Design review of the part built by this model. Coordinates are the model's own, in mm. Coordinates: 2 decimals unless noted, no trailing zeros. Write each loop counter-clockwise with the first axis right and the second up, starting at its lowest first coordinate (ties: lowest second). Pieces come first, ordered by that corner, then holes. Notation, with made-up numbers: (65, 23.25) - (79, 23.25) arc R16 ccw to (79, 40.25) - close; hole circle Ø7 at (33.5, 69). An arc over 180 degrees is marked (long way). Use a Markdown table: item, result.
Autodesk Inventor part; units mm, degrees
ref_plane "tuer_XY" through (241.2, -320.6, -8.2) normal (0, 1, 0) x (1, 0, 0)
ref_plane "tuer_YZ" through (241.2, -320.6, -8.2) normal (1, 0, 0) x (0, 0, -1)
ref_plane "tuer_ZX" through (241.2, -320.6, -8.2) normal (0, 0, -1) x (0, 1, 0)
sketch "Skizze_1" plane through (0, 0, 0) normal (0, 0, 1) x (1, 0, 0)
  line L0 (-247.5, 377.5) -> (-247.5, -377.5)
  line L1 (-247.5, -377.5) -> (247.5, -377.5)
  line L2 (247.5, -377.5) -> (247.5, 377.5)
  line L3 (247.5, 377.5) -> (-247.5, 377.5)
extrude "Extrusion1" add sketch "Skizze_1" against normal blind 15
sketch "Skizze_2" plane through (0, 0, 0) normal (1, 0, 0) x (0, 0, -1)
  line L0 (2, 375.5) -> (2, -375.5)
  line L1 (2, -375.5) -> (17, -375.5)
  line L2 (17, -375.5) -> (17, 375.5)
  line L3 (17, 375.5) -> (2, 375.5)
extrude "Extrusion2" cut sketch "Skizze_2" along normal mid plane 491
sketch "Skizze_3" plane through (0, 0, -2) normal (0, 0, 1) x (1, 0, 0)
  line L0 (-245.5, 361.5) -> (231.5, 361.5)
  line L1 (231.5, 361.5) -> (231.5, -361.5)
  line L2 (231.5, -361.5) -> (-245.5, -361.5)
  line L3 (-245.5, -361.5) -> (-245.5, -373.5)
  line L4 (-245.5, -373.5) -> (243.5, -373.5)
  line L5 (243.5, -373.5) -> (243.5, 373.5)
  line L6 (243.5, 373.5) -> (-245.5, 373.5)
  line L7 (-245.5, 373.5) -> (-245.5, 361.5)
sketch "Skizze_21" plane through (0, -320.6, 0) normal (0, 1, 0) x (1, 0, 0)
  arc A0 (241.2, 12.35) -> (241.2, 4.05) centre (241.2, 8.2) ccw
  line L0 (241.2, 4.05) -> (245.5, 4.05)
  line L1 (245.5, 4.05) -> (245.5, 5.5)
  line L2 (245.5, 5.5) -> (241.2, 5.5)
  arc A1 (241.2, 10.9) -> (241.2, 5.5) centre (241.2, 8.2) ccw
  line L3 (241.2, 10.9) -> (245.5, 10.9)
  line L4 (245.5, 10.9) -> (245.5, 12.35)
  line L5 (245.5, 12.35) -> (241.2, 12.35)
extrude "Extrusion3" add sketch "Skizze_21" along normal mid plane 26
sketch "Skizze_22" plane through (0, 320.6, 0) normal (0, 1, 0) x (1, 0, 0)
  arc A0 (241.2, 12.35) -> (241.2, 4.05) centre (241.2, 8.2) ccw
  line L0 (241.2, 4.05) -> (245.5, 4.05)
  line L1 (245.5, 4.05) -> (245.5, 5.5)
  line L2 (245.5, 5.5) -> (241.2, 5.5)
  arc A1 (241.2, 10.9) -> (241.2, 5.5) centre (241.2, 8.2) ccw
  line L3 (241.2, 10.9) -> (245.5, 10.9)
  line L4 (245.5, 10.9) -> (245.5, 12.35)
  line L5 (245.5, 12.35) -> (241.2, 12.35)
extrude "Extrusion4" add sketch "Skizze_22" along normal mid plane 26
sketch "Skizze_24" plane through (0, 0, 0) normal (0, 0, 1) x (1, 0, 0)
  line L0 (-221.05, -318.95) -> (-221.05, -341.05)
  line L1 (-221.05, -341.05) -> (-198.95, -341.05)
  line L2 (-198.95, -341.05) -> (-198.95, -318.95)
  line L3 (-198.95, -318.95) -> (-221.05, -318.95)
extrude "Extrusion5" cut sketch "Skizze_24" against normal blind 2
sketch "Skizze_41" plane through (0, 0, 0) normal (0, 0, 1) x (1, 0, 0)
  line L0 (-221.05, 341.05) -> (-221.05, 318.95)
  line L1 (-221.05, 318.95) -> (-198.95, 318.95)
  line L2 (-198.95, 318.95) -> (-198.95, 341.05)
  line L3 (-198.95, 341.05) -> (-221.05, 341.05)
extrude "Extrusion6" cut sketch "Skizze_41" against normal blind 2
sketch "Skizze_23" plane through (-247.5, 0, 0) normal (1, 0, 0) x (0, 0, -1)
  arc A0 (13.25, 372.2142) -> (13.25, 354.7858) centre (15.5, 363.5) ccw
  arc A1 (15.5, 351.881) -> (13.25, 354.7858) centre (12.5, 351.881) ccw
  line L0 (15.5, 351.881) -> (15.5, 375.119)
  arc A2 (13.25, 372.2142) -> (15.5, 375.119) centre (12.5, 375.119) ccw
extrude "Extrusion7" cut sketch "Skizze_23" along normal blind 3
sketch "Skizze_26" plane through (-247.5, 0, 0) normal (1, 0, 0) x (0, 0, -1)
  arc A0 (13.25, -354.7858) -> (13.25, -372.2142) centre (15.5, -363.5) ccw
  arc A1 (15.5, -375.119) -> (13.25, -372.2142) centre (12.5, -375.119) ccw
  line L0 (15.5, -375.119) -> (15.5, -351.881)
  arc A2 (13.25, -354.7858) -> (15.5, -351.881) centre (12.5, -351.881) ccw
extrude "Extrusion8" cut sketch "Skizze_26" along normal blind 3
extrude "Extrusion9" add sketch "Skizze_3" against normal blind 6.5
ref_plane "tuer_XY" through (241.2, -320.6, -8.2) normal (0, 1, 0) x (1, 0, 0)
ref_plane "tuer_YZ" through (241.2, -320.6, -8.2) normal (1, 0, 0) x (0, 0, -1)
ref_plane "tuer_ZX" through (241.2, -320.6, -8.2) normal (0, 0, -1) x (0, 1, 0)
ref_plane "verschluss_XY" through (-210, -330, 0) normal (0, 0, 1) x (1, 0, 0)
ref_plane "verschluss_YZ" through (-210, -330, 0) normal (1, 0, 0) x (0, 1, 0)
ref_plane "verschluss_ZX" through (-210, -330, 0) normal (0, 1, 0) x (0, 0, 1)
ref_plane "verschluss2_XY" through (-210, 330, 0) normal (0, 0, 1) x (1, 0, 0)
ref_plane "verschluss2_YZ" through (-210, 330, 0) normal (1, 0, 0) x (0, 1, 0)
ref_plane "verschluss2_ZX" through (-210, 330, 0) normal (0, 1, 0) x (0, 0, 1)
sketch "Эскиз10" plane through (0, 0, 0) normal (0, 0, 1) x (1, 0, 0)
  line L0 (-39.5, 292.5) -> (52.5, 292.5)
  line L1 (52.5, 292.5) -> (52.5, 200.5)
  line L2 (52.5, 200.5) -> (-39.5, 200.5)
  line L3 (-39.5, 200.5) -> (-39.5, 292.5)
  line L4 (247.5, -377.5) -> (247.5, 377.5)
  line L5 (247.5, 377.5) -> (-247.5, 377.5)
  point P0 (0, 0)
  dimension "d20" = 92
  dimension "d21" = 92
  dimension "d22" = 195
  dimension "d23" = 85
extrude "Выдавливание10" cut sketch "Эскиз10" against normal blind 10
properties part number "1130_01_03 (2)"
(1) For pin 1 (4 mm diameter, centred on x = 147, y = 268.5, fed in from -Z), flat-tipped, find the tip position at first contact; note if it passes through.
Determined:
| item | result |
|---|---|
| pin 1 | z = -2 |
(2) Take a section at B-B on y = -123.5. Write out the cut boundary in (x, z).
Determined:
| item | result |
|---|---|
| outline | (-247.5, -15) - (-245.5, -15) - (-245.5, -2) - (231.5, -2) - (231.5, -8.5) - (243.5, -8.5) - (243.5, -2) - (245.5, -2) - (245.5, -15) - (247.5, -15) - (247.5, 0) - (-247.5, 0) - close |
(3) Draft analysis for pull direction Y (two halves, no side actions). For faces 1 (the flat face through (3, 377.5, -7)), 2 (the flat face through (-10, 5, -2)), 3 (the flat face through (-3, -377.5, -7)), 4 (the flat face through (-3, 5, 0)), state which applies: +Y half, -Y half, draft (parallel to the pull), parting line (faces both ways), or undercut.
Determined:
| item | result |
|---|---|
| face 1 | +Y half |
| face 2 | undercut |
| face 3 | -Y half |
| face 4 | draft |
(4) For L1, parallel to Y at x = 114, z = -8; L2, parallel to X at y = 300, z = -6.5; L3, parallel to X at y = 86.5, z = -9.75, list the stretches that pass through material, from the lowest coordinate up. Write a range as from..to.
Determined:
| item | result |
|---|---|
| L1 | -377.5..-375.5, -373.5..-361.5, 361.5..373.5, 375.5..377.5 |
| L2 | -247.5..-245.5, 231.5..243.5, 245.5..247.5 |
| L3 | -247.5..-245.5, 245.5..247.5 |
(5) Take a section at A-A on x = 33.5. Write out the cut boundary in (y, z).
Determined:
| item | result |
|---|---|
| outline | (-377.5, -15) - (-375.5, -15) - (-375.5, -2) - (-373.5, -2) - (-373.5, -8.5) - (-361.5, -8.5) - (-361.5, -2) - (200.5, -2) - (200.5, 0) - (-377.5, 0) - close; (292.5, -2) - (361.5, -2) - (361.5, -8.5) - (373.5, -8.5) - (373.5, -2) - (375.5, -2) - (375.5, -15) - (377.5, -15) - (377.5, 0) - (292.5, 0) - close |
(6) Take a section at C-C on x = 191.5. Write out the cut boundary in (y, z), and give its area (3 significant figures).
Determined:
| item | result |
|---|---|
| outline | (-377.5, -15) - (-375.5, -15) - (-375.5, -2) - (-373.5, -2) - (-373.5, -8.5) - (-361.5, -8.5) - (-361.5, -2) - (361.5, -2) - (361.5, -8.5) - (373.5, -8.5) - (373.5, -2) - (375.5, -2) - (375.5, -15) - (377.5, -15) - (377.5, 0) - (-377.5, 0) - close |
| area | 1,720 mm2 |
